```python
from build123d import *

# Parameters (mm, degrees)
ESQUISSE1_R             = 35
EXTRUSION1_DEPTH        = 24
CONG_1_R                = 12
CONG_2_R                = 12
ESQUISSE2_R             = 19
ENL_V_MAT_EXTRU_1_DEPTH = 7
ENL_V_START             = -7
ESQUISSE3_R             = 19
ENL_V_MAT_EXTRU_2_DEPTH = 7
ESQUISSE5_R             = 9.5
ESQUISSE5_R_2           = 2
ENL_V_MAT_EXTRU_3_DEPTH = 53.335456499


with BuildPart() as part:
    # Esquisse1 → Extrusion1 (new body)
    with BuildSketch(Plane.XY):
        Circle(ESQUISSE1_R)
    extrude(amount=EXTRUSION1_DEPTH)

    # Congé1
    cong_1_edges = [part.edges().sort_by_distance(p)[0] for p in [
        (-35, 0, 24),
    ]]
    fillet(cong_1_edges, radius=CONG_1_R)

    # Congé2
    cong_2_edges = [part.edges().sort_by_distance(p)[0] for p in [
        (-35, 0, 0),
    ]]
    fillet(cong_2_edges, radius=CONG_2_R - 0.0001)  # a hair under: the kernel refuses the full size

    # Esquisse2 → Enlèv. mat.-Extru.1 (cut)
    with BuildSketch(Plane.XY.offset(24)):
        Circle(ESQUISSE2_R)
    extrude(amount=-ENL_V_MAT_EXTRU_1_DEPTH, mode=Mode.SUBTRACT)

    # Esquisse3 → Enlèv. mat.-Extru.2 (cut)
    with BuildSketch(Plane(origin=(0, 0, 0), x_dir=(-1, 0, 0), z_dir=(0, 0, -1)).offset(ENL_V_START)):
        with Locations(Location((0, 0, 0), (0, 0, 180))):
            Circle(ESQUISSE3_R)
    extrude(amount=ENL_V_MAT_EXTRU_2_DEPTH, mode=Mode.SUBTRACT)

    # Esquisse5 → Enlèv. mat.-Extru.3 (cut, through all)
    with BuildSketch(Plane.XY.offset(17)):
        Circle(ESQUISSE5_R)
        with Locations((0, 14.25)):
            Circle(ESQUISSE5_R_2)
        with Locations((12.340862004, -7.125)):
            Circle(ESQUISSE5_R_2)
        with Locations((-12.340862004, -7.125)):
            Circle(ESQUISSE5_R_2)
    extrude(amount=-ENL_V_MAT_EXTRU_3_DEPTH, mode=Mode.SUBTRACT)


solid = part.part
```
Model file for the job. Use its own axes, mm. A direction names the side the tool comes from. Coordinates: 2 decimals unless noted, no trailing zeros. Order: outer loops, then holes, each group sorted by start corner. A loop starts at its lowest first (then second) coordinate and runs counter-clockwise, first axis right, second up. Notation, with made-up numbers: (-37.5, 51) -> (13.5, 51) arc R17 cw to (13.5, 77) -> close; hole circle Ø9 at (44, 38). An arc over 180 degrees is marked (long way). Answer as a JSON object with one key per item and string values. Group by question number.
1) Which spindle directions (+Z, -Z, +X, -X, +Y, -Y) get a long thin tool onto all of the face, cutting with end or side? Do faces 1 (the face through (8.767, -16.856, 20.549)), 2 (the face through (-14.34, -7.04, 12.07)), 3 (the face through (-4.119, 18.548, 3.549)). Say none if no direction does.
2) Cut at C-C, the plane z = 13.25. Write the cut outline in (x, y) (3 decimals), then the cut area to 3 significant figures.
3) Pull direction Y, two halves, no side cores. Call faces 4 (the face through (3, 19, 0)), 5 (the face through (4.38, -8.43, 12.07)): +Y half, -Y half, draft (parallel to the pull), parting line (faces both ways), or undercut.
4) Cut at A-A, the plane x = 0. Count the separate pieces of the cut face and the enclosed holes in it, then the cut area to 3 significant figures.
5) Flat gauge pins, fed straight in: pin 1 (1.5 mm diameter, centred on x = 0, y = 15, fed in from -Z); pin 2 (12 mm diameter, centred on x = 13.5, z = 3.5, fed in from +Y); pin 3 (6 mm diameter, centred on y = -1.5, z = 16.5, fed in from +X); pin 4 (6.5 mm diameter, centred on x = 0, y = 14.25, fed in from -Z). Where does each tip first touch, or does it go through?
6) Drill centre lines: L1, parallel to Y at x = 0, z = 9.75; L2, parallel to Y at x = 0, z = 9.25; L3, parallel to Z at x = 5, y = -10. Where is each one in solid material? Low to high.
7) Cut at D-D, the plane z = 1.75. Write the cut outline in (x, y).
Check values:
{
 "1": {"face 1": "+Z", "face 2": "+Z, -Z", "face 3": "-Z"},
 "2": {"outline": "circle Ø69.869 at (0, 0); hole circle Ø4 at (-12.341, -7.125); hole circle Ø19 at (0, 0); hole circle Ø4 at (0, 14.25); hole circle Ø4 at (12.341, -7.125)", "area": "3,510 mm²"},
 "3": {"face 4": "draft", "face 5": "undercut"},
 "4": {"separate pieces": "3", "enclosed holes": "0", "area": "794 mm²"},
 "5": {"pin 1": "passes through", "pin 2": "stops at y = 32.97", "pin 3": "stops at x = 34.89", "pin 4": "stops at z = 7"},
 "6": {"L1": "y = -34.79 to -9.5, 9.5 to 12.25, 16.25 to 34.79", "L2": "y = -34.68 to -9.5, 9.5 to 12.25, 16.25 to 34.68", "L3": "z = 7 to 17"},
 "7": {"outline": "circle Ø58.48 at (0, 0); hole circle Ø38 at (0, 0)"}
}
